from build123d import *

# Parameters (mm, degrees)
BOSS_EXTRUDE6_DEPTH      = 2.9
SKETCH27_R               = 1.05
CUT_EXTRUDE12_DEPTH      = 3.9
SKETCH29_W               = 20
SKETCH29_H               = 4.356134153
BOSS_EXTRUDE8_DEPTH      = 11.5
BOSS_EXTRUDE8_DEPTH_BACK = 2.9
CUT_EXTRUDE16_DEPTH      = 24.656134153
SKETCH34_R               = 1
CUT_EXTRUDE17_DEPTH      = 11.4
CUT_EXTRUDE18_DEPTH      = 3.9
FILLET1_R                = 5
FILLET1_OF_MIRROR1_R     = 5


with BuildPart() as part:
    # Sketch26 → Boss-Extrude6 (new body)
    with BuildSketch(Plane(origin=(0, 0, 0), x_dir=(1, 0, 0), z_dir=(0, 1, 0))):
        with BuildLine():
            Line((-13.656134153, -7.7), (-13.656134153, 7.7))
            ThreePointArc((-13.656134153, 7.7), (0, 21.356134153), (13.656134153, 7.7))
            Line((13.656134153, 7.7), (13.656134153, -7.7))
            ThreePointArc((13.656134153, -7.7), (0, -21.356134153), (-13.656134153, -7.7))
        make_face()
        with BuildLine():
            Line((-8.5, 7.7), (-8.5, -7.7))
            ThreePointArc((-8.5, -7.7), (0, -16.2), (8.5, -7.7))
            Line((8.5, -7.7), (8.5, 7.7))
            ThreePointArc((8.5, 7.7), (0, 16.2), (-8.5, 7.7))
        make_face(mode=Mode.SUBTRACT)
    extrude(amount=BOSS_EXTRUDE6_DEPTH)

    # Sketch27 → Cut-Extrude12 (cut, through all)
    with BuildSketch(Plane(origin=(0, 2.9, 0), x_dir=(1, 0, 0), z_dir=(0, 1, 0))):
        with Locations((-8, 15)):
            Circle(SKETCH27_R)
        with Locations((8, 15)):
            Circle(SKETCH27_R)
        with Locations((8, -15)):
            Circle(SKETCH27_R)
        with Locations((-8, -15)):
            Circle(SKETCH27_R)
    extrude(amount=-CUT_EXTRUDE12_DEPTH, mode=Mode.SUBTRACT)

    # Sketch29 → Boss-Extrude8 (add, two sides)
    with BuildSketch(Plane(origin=(0, 2.9, 0), x_dir=(1, 0, 0), z_dir=(0, 1, 0))) as boss_extrude8_sk:
        with Locations((0, -19.178067076)):
            Rectangle(SKETCH29_W, SKETCH29_H)
    extrude(amount=BOSS_EXTRUDE8_DEPTH)
    extrude(boss_extrude8_sk.sketch, amount=-BOSS_EXTRUDE8_DEPTH_BACK)

    # Sketch33 → Cut-Extrude16 (cut, through all)
    with BuildSketch(Plane(origin=(10, 0, 0), x_dir=(0, 0, -1), z_dir=(1, 0, 0))):
        Polygon((-21.356134153, 14.4), (-21.356134153, 10.4), (-17, 7.884984774), (-17, 14.4), align=None)
    extrude(amount=-CUT_EXTRUDE16_DEPTH, mode=Mode.SUBTRACT)

    # Sketch34 → Cut-Extrude17 (cut, through all)
    with BuildSketch(Plane.XZ):
        with Locations((6.5, 19)):
            Circle(SKETCH34_R)
        with Locations((-6.5, 19)):
            Circle(SKETCH34_R)
    extrude(amount=-CUT_EXTRUDE17_DEPTH, mode=Mode.SUBTRACT)

    # Sketch35 → Cut-Extrude18 (cut, through all)
    with BuildSketch(Plane(origin=(0, 2.9, 0), x_dir=(1, 0, 0), z_dir=(0, 1, 0))):
        Polygon((-10, 9.72081528), (-10, -9.72081528), (-6.01040764, -13.71040764), (-6.01040764, 13.71040764), align=None)
    cut_extrude18 = extrude(amount=-CUT_EXTRUDE18_DEPTH, mode=Mode.SUBTRACT)

    # Fillet1
    fillet1_edges = [part.edges().sort_by_distance(p)[0] for p in [
        (-10, 1.45, -9.72081528),
        (-10, 1.45, 9.72081528),
    ]]
    fillet(fillet1_edges, radius=FILLET1_R)

    # Mirror1: Cut-Extrude18 across plane
    add(cut_extrude18.mirror(Plane(origin=(0, 0, 0), x_dir=(0, 0, 1), z_dir=(1, 0, 0))), mode=Mode.SUBTRACT)

    # Fillet1 of Mirror1
    fillet1_of_mirror1_edges = [part.edges().sort_by_distance(p)[0] for p in [
        (10, 1.45, -9.72081528),
        (10, 1.45, 9.72081528),
    ]]
    fillet(fillet1_of_mirror1_edges, radius=FILLET1_OF_MIRROR1_R)


solid = part.part
Could you check a few things on this model? Use its own coordinates, in mm. A direction names the side the tool comes from. Give positions to 0.01 mm unless a question says otherwise; leave off trailing zeros. Order: outer loops, then holes, each group sorted by start corner. A loop starts at its lowest first (then second) coordinate and runs counter-clockwise, first axis right, second up. Notation, with made-up numbers: (-33.75, 66.25) -> (9.25, 66.25) arc R7 ccw to (9.25, 76.25) -> close; hole circle Ø9 at (-9, 22). An arc over 180 degrees is marked (long way). Return JSON: item names as keys, results as strings.
1. Imagine slicing it at C-C on z = 1. List the corners of the cut face in (x, y) for me, then the cut area to 3 significant figures.
Answer list:
{"outline": "(-13.66, 0) -> (-10, 0) -> (-10, 2.9) -> (-13.66, 2.9) -> close; (10, 0) -> (13.66, 0) -> (13.66, 2.9) -> (10, 2.9) -> close", "area": "21.2 mm2"}
2. Thinking about a two-plate mould opening in Z: for faces 4 (the flat face through (0, 5, 21.356)), 5 (the flat face through (10, 5, 19)), 6 (the cylindrical face through (9.61, 1.43, 9.59)), which applies, pulls with the +Z half, pulls with the -Z half, needs draft (parallel to the pull), parting line crosses it, or undercut?
Answer list:
{"face 4": "pulls with the +Z half", "face 5": "needs draft", "face 6": "undercut"}
3. On a 3-axis mill with a long thin cutter (end or side, diameter ignored), from which of +Z, -Z, +X, -X, +Y, -Y can I reach the whole of each face in a straight line? I mean faces 1 (the flat face through (10.2, 2.9, -2.3)), 2 (the flat face through (-10.2, 0, -1.7)), 3 (the flat face through (7.255, 1.47, -12.466)). Say none if no direction works.
Answer list:
{"face 1": "-Z, +X, -X, +Y", "face 2": "+Z, -Z, +X, -X, -Y", "face 3": "+Y, -Y"}
4. For pin 1 Ø1 at (x, z) = (-8.5, 6.5) entering from +Y; pin 2 Ø5 at (y, z) = (6, 19) entering from -X; pin 3 Ø1 at (x, z) = (-10, -3.5) entering from +Y; pin 4 Ø4 at (y, z) = (4, -11.5) entering from +X, each with a flat end and sliding along its axis, tell me the tip position at first contact or that it passes through.
Answer list:
{"pin 1": "passes through", "pin 2": "stops at x = -10", "pin 3": "stops at y = 2.9", "pin 4": "stops at x = 13.49"}
5. Imagine slicing it at A-A on y = 1.75. List the corners of the cut face in (x, z) for me, then the cut area to 3 significant figures.
Answer list:
{"outline": "(-13.66, -7.7) arc R13.66 ccw to (13.66, -7.7) -> (13.66, 7.7) arc R13.66 ccw to (10, 17) -> (10, 21.36) -> (-10, 21.36) -> (-10, 17) arc R13.66 ccw to (-13.66, 7.7) -> close; hole (-10, -7.65) arc R5 ccw to (-8.54, -11.19) -> (-6.01, -13.71) arc R8.5 ccw to (6.01, -13.71) -> (8.54, -11.19) arc R5 ccw to (10, -7.65) -> (10, 7.65) arc R5 ccw to (8.54, 11.19) -> (6.01, 13.71) arc R8.5 ccw to (-6.01, 13.71) -> (-8.54, 11.19) arc R5 ccw to (-10, 7.65) -> close; hole circle Ø2.1 at (-8, -15); hole circle Ø2.1 at (-8, 15); hole circle Ø2 at (-6.5, 19); hole circle Ø2 at (6.5, 19); hole circle Ø2.1 at (8, -15); hole circle Ø2.1 at (8, 15)", "area": "458 mm2"}
6. Imagine slicing it at B-B on x = 8. List the corners of the cut face in (y, z) for me.
Answer list:
{"outline": "(0, -18.77) -> (2.9, -18.77) -> (2.9, -16.05) -> (0, -16.05) -> close; (0, -13.95) -> (2.9, -13.95) -> (2.9, -11.72) -> (0, -11.72) -> close; (0, 11.72) -> (2.9, 11.72) -> (2.9, 13.95) -> (0, 13.95) -> close; (0, 16.05) -> (2.9, 16.05) -> (2.9, 17) -> (7.88, 17) -> (10.4, 21.36) -> (0, 21.36) -> close"}
7. I need wall thicknesses on line 1 (X direction, y = 6, z = 19); line 2 (X direction, y = 2.15, z = 15); line 3 (Z direction, x = 6.5, y = 4.5). Which ranges of each line are inside material? Lowest first, please. Write a range as from..to.
Answer list:
{"line 1": "x = -10..-7.5, -5.5..5.5, 7.5..10", "line 2": "x = -11.54..-9.05, -6.95..-4.35, 4.35..6.95, 9.05..11.54", "line 3": "z = 17..18, 20..21.36"}
8. Imagine slicing it at D-D on z = 19. List the corners of the cut face in (x, y) for me, then the cut area to 3 significant figures.
Answer list:
{"outline": "(-10, 0) -> (-7.5, 0) -> (-7.5, 9.04) -> (-10, 9.04) -> close; (-5.5, 0) -> (5.5, 0) -> (5.5, 9.04) -> (-5.5, 9.04) -> close; (7.5, 0) -> (10, 0) -> (10, 9.04) -> (7.5, 9.04) -> close", "area": "145 mm2"}
